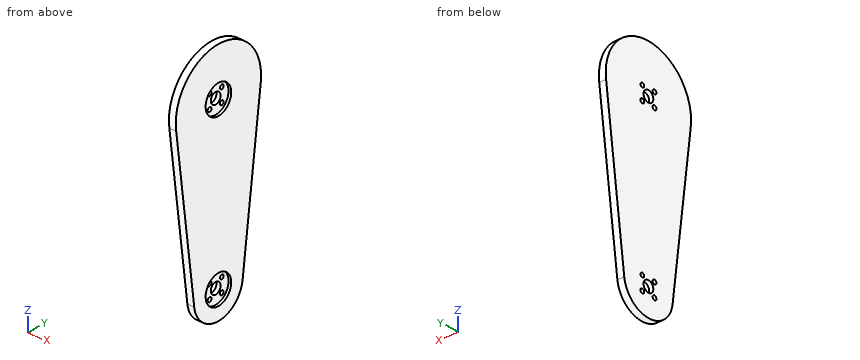
from build123d import *

# Parameters (mm, degrees)
SKETCH_1_R          = 1.55
SKETCH_1_R_2        = 4
EXTRUDE_3_DEPTH     = 5
SKETCH_3_R          = 10.5
CUT_EXTRUDE_2_DEPTH = 2


with BuildPart() as part:
    # 草图1 → 凸台-拉伸3 (new body)
    with BuildSketch(Plane(origin=(0, 0, 0), x_dir=(0, 0, -1), z_dir=(1, 0, 0))):
        with BuildLine():
            Line((122.5, 19.843134833), (4.375, 34.725485958))
            ThreePointArc((4.375, 34.725485958), (-34.998579399, -0.315341144), (5, -34.641016151))
            Line((5, -34.641016151), (122.499047902, -19.843254763))
            ThreePointArc((122.499047902, -19.843254763), (139.999999994, -0.000479811), (122.5, 19.843134833))
        make_face()
        with Locations((-5, -5)):
            Circle(SKETCH_1_R, mode=Mode.SUBTRACT)
        with Locations((5, -5)):
            Circle(SKETCH_1_R, mode=Mode.SUBTRACT)
        with Locations((-5, 5)):
            Circle(SKETCH_1_R, mode=Mode.SUBTRACT)
        Circle(SKETCH_1_R_2, mode=Mode.SUBTRACT)
        with Locations((5, 5)):
            Circle(SKETCH_1_R, mode=Mode.SUBTRACT)
        with Locations((115, -5)):
            Circle(SKETCH_1_R, mode=Mode.SUBTRACT)
        with Locations((125, -5)):
            Circle(SKETCH_1_R, mode=Mode.SUBTRACT)
        with Locations((125, 5)):
            Circle(SKETCH_1_R, mode=Mode.SUBTRACT)
        with Locations((115, 5)):
            Circle(SKETCH_1_R, mode=Mode.SUBTRACT)
        with Locations((120, 0)):
            Circle(SKETCH_1_R_2, mode=Mode.SUBTRACT)
    extrude(amount=EXTRUDE_3_DEPTH)

    # 草图3 → 切除-拉伸2 (cut)
    with BuildSketch(Plane(origin=(5, 0, 0), x_dir=(0, 0, -1), z_dir=(1, 0, 0))):
        Circle(SKETCH_3_R)
        with Locations((120, 0)):
            Circle(SKETCH_3_R)
    extrude(amount=-CUT_EXTRUDE_2_DEPTH, mode=Mode.SUBTRACT)


solid = part.part
The model under review builds one solid part; all positions refer to its coordinate system, in mm. Round coordinates to 2 decimals unless told otherwise and drop trailing zeros. Order: outer loops, then holes, each group sorted by start corner. A loop starts at its lowest first (then second) coordinate and runs counter-clockwise, first axis right, second up. Notation, with made-up numbers: (8.25, 78.25) -> (42.25, 78.25) arc R16 ccw to (42.25, 104.25) -> close; hole circle Ø4 at (-36.5, 25.5). An arc over 180 degrees is marked (long way). Write item = value, one per line. Start each with the question number.
Item 1: For line 1 along Z through (x, y) = (2.1, 0); line 2 along Y through (x, z) = (1.15, -125); line 3 along Y through (x, z) = (1.8, 0), list the stretches that pass through material, from the lowest coordinate up.
Item 2: Clearance check with flat-ended pins moving along their axes: pin 1 Ø1 at (x, y) = (0.5, -14) entering from +Z; pin 2 Ø17 at (y, z) = (0, -120) entering from +X; pin 3 Ø1 at (x, y) = (1, -11) entering from -Z; pin 4 Ø23 at (y, z) = (1, 1.5) entering from +X. State where each tip first meets the part, or that it passes through.
Item 3: Consider section B-B on x = 1.65. Count the separate pieces of the cut face and the enclosed holes in it, plus the area to 3 significant figures.
Item 4: Consider section A-A on y = 0. Write out the cut boundary in (x, z), plus the area to 3 significant figures.
Item 5: Consider section C-C on z = -120. Write out the cut boundary in (x, y), plus the area to 3 significant figures.
Item 6: Consider section D-D on z = -60. Write out the cut boundary in (x, y).
Conclusion:
q1.line_1 = -140 to -124, -116 to -4, 4 to 35
q1.line_2 = -19.36 to -6.55, -3.45 to 3.45, 6.55 to 19.36
q1.line_3 = -35 to -4, 4 to 35
q2.pin_1 = 32.29
q2.pin_2 = 3
q2.pin_3 = -137.02
q2.pin_4 = 5
q3.separate_pieces = 1
q3.enclosed_holes = 10
q3.area = 9,040 mm2
q4.outline = (0, -140) -> (5, -140) -> (5, -130.5) -> (3, -130.5) -> (3, -124) -> (0, -124) -> close; (0, -116) -> (3, -116) -> (3, -109.5) -> (5, -109.5) -> (5, -10.5) -> (3, -10.5) -> (3, -4) -> (0, -4) -> close; (0, 4) -> (3, 4) -> (3, 10.5) -> (5, 10.5) -> (5, 35) -> (0, 35) -> close
q4.area = 743 mm2
q5.outline = (0, -20.16) -> (5, -20.16) -> (5, -10.5) -> (3, -10.5) -> (3, -4) -> (0, -4) -> close; (0, 4) -> (3, 4) -> (3, 10.5) -> (5, 10.5) -> (5, 20.16) -> (0, 20.16) -> close
q5.area = 136 mm2
q6.outline = (0, -27.71) -> (5, -27.71) -> (5, 27.72) -> (0, 27.72) -> close
